from build123d import *

# Parameters (mm, degrees)
CHANFREIN1_SIZE                                = 0.5
FRAISAGE_POUR_VIS_T_TE_FRAIS_E_M31_D           = 3.2
FRAISAGE_POUR_VIS_T_TE_FRAIS_E_M31_CSINK_D     = 7.3
FRAISAGE_POUR_VIS_T_TE_FRAIS_E_M31_CSINK_ANGLE = 90
ENL_V_MAT_EXTRU_1_REACH                        = 94.326
ESQUISSE5_R                                    = 2.5


with BuildPart() as part:
    # Esquisse1 → Révolution1 (revolve)
    with BuildSketch(Plane.XY, mode=Mode.PRIVATE) as r_volution1_sk:
        Polygon((0, 10), (0, 20), (78, 20), (78, 30), (82, 30), (82, 17), (4, 17), (4, 10), align=None)
    revolve(r_volution1_sk.sketch.rotate(Axis((0, 0, 0), (1, 0, 0)), 90), axis=Axis((0, 0, 0), (1, 0, 0)))

    # Chanfrein1
    chanfrein1_edges = [part.edges().sort_by_distance(p)[0] for p in [
        (0, 0, -20),
        (78, 0, -30),
        (82, 0, -30),
        (82, 0, -17),
        (4, 0, -10),
    ]]
    chamfer(chanfrein1_edges, length=CHANFREIN1_SIZE)

    # Fraisage pour vis à tête fraisée M31 (through all)
    with Locations(Plane.ZY):
        with Locations((0, 13), (13, 0), (0, -13), (-13, 0)):
            CounterSinkHole(FRAISAGE_POUR_VIS_T_TE_FRAIS_E_M31_D / 2, FRAISAGE_POUR_VIS_T_TE_FRAIS_E_M31_CSINK_D / 2, counter_sink_angle=FRAISAGE_POUR_VIS_T_TE_FRAIS_E_M31_CSINK_ANGLE)

    # Esquisse5 → Enlèv. mat.-Extru.1 (cut, up to next)
    with BuildSketch(Plane(origin=(82, 0, 0), x_dir=(0, 0, -1), z_dir=(1, 0, 0)), mode=Mode.PRIVATE) as enl_v_mat_extru_1_sk1:
        with Locations((0, 25)):
            Circle(ESQUISSE5_R)
    enl_v_mat_extru_1_tool1 = extrude(enl_v_mat_extru_1_sk1.sketch, amount=-ENL_V_MAT_EXTRU_1_REACH, mode=Mode.PRIVATE) & part.part
    # Esquisse5 → Enlèv. mat.-Extru.1 (cut, up to next)
    with BuildSketch(Plane(origin=(82, 0, 0), x_dir=(0, 0, -1), z_dir=(1, 0, 0)), mode=Mode.PRIVATE) as enl_v_mat_extru_1_sk2:
        with Locations((25, 0)):
            Circle(ESQUISSE5_R)
    enl_v_mat_extru_1_tool2 = extrude(enl_v_mat_extru_1_sk2.sketch, amount=-ENL_V_MAT_EXTRU_1_REACH, mode=Mode.PRIVATE) & part.part
    # Esquisse5 → Enlèv. mat.-Extru.1 (cut, up to next)
    with BuildSketch(Plane(origin=(82, 0, 0), x_dir=(0, 0, -1), z_dir=(1, 0, 0)), mode=Mode.PRIVATE) as enl_v_mat_extru_1_sk3:
        with Locations((-25, 0)):
            Circle(ESQUISSE5_R)
    enl_v_mat_extru_1_tool3 = extrude(enl_v_mat_extru_1_sk3.sketch, amount=-ENL_V_MAT_EXTRU_1_REACH, mode=Mode.PRIVATE) & part.part
    # Esquisse5 → Enlèv. mat.-Extru.1 (cut, up to next)
    with BuildSketch(Plane(origin=(82, 0, 0), x_dir=(0, 0, -1), z_dir=(1, 0, 0)), mode=Mode.PRIVATE) as enl_v_mat_extru_1_sk4:
        with Locations((0, -25)):
            Circle(ESQUISSE5_R)
    enl_v_mat_extru_1_tool4 = extrude(enl_v_mat_extru_1_sk4.sketch, amount=-ENL_V_MAT_EXTRU_1_REACH, mode=Mode.PRIVATE) & part.part
    add(enl_v_mat_extru_1_tool1.solids().sort_by_distance((82, 25, 0))[0], mode=Mode.SUBTRACT)
    add(enl_v_mat_extru_1_tool2.solids().sort_by_distance((82, 0, -25))[0], mode=Mode.SUBTRACT)
    add(enl_v_mat_extru_1_tool3.solids().sort_by_distance((82, 0, 25))[0], mode=Mode.SUBTRACT)
    add(enl_v_mat_extru_1_tool4.solids().sort_by_distance((82, -25, 0))[0], mode=Mode.SUBTRACT)


solid = part.part
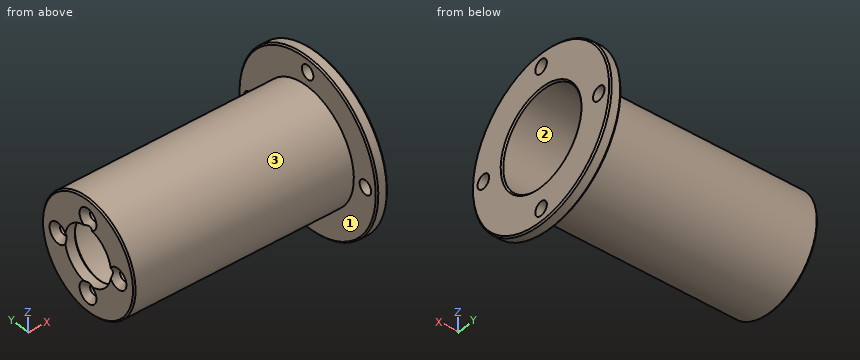
Here's how the part is built. I have some questions about the finished solid (model axes, mm). Face numbers are marked on the shaded views. Coordinates: 2 decimals unless noted, no trailing zeros. Loops run counter-clockwise (first coordinate to the right, second up) from the corner with the lowest first, then second, coordinate; pieces in that order, holes last.
1. I need wall thicknesses on L1, parallel to Y at x = 2, z = 0; L2, parallel to Y at x = 53, z = 0; L3, parallel to Y at x = 61, z = -9.5. Which ranges of each line are inside material? Lowest first, please.
2. If we mould it in two halves opening along Y, with no side actions, what happens to the marked faces 1, 2 and 3? For each: pulls with the +Y half, pulls with the -Y half, needs draft (parallel to the pull), parting line crosses it, or undercut.
3. Imagine slicing it at A-A, the plane z = 0. Count the separate pieces of the cut face and the enclosed holes in it, and give its area (3 significant figures).
4. Imagine slicing it at C-C, the plane x = 11. Please give me the cut outline in (y, z), and give its area (3 significant figures).
5. For P1, Ø5, axis at x = 28, z = 9.5, coming from the +Y side (3 decimals); P2, Ø3, axis at y = 25, z = 0, coming from the +X side; P3, Ø6, axis at x = 61, z = -20.5, coming from the -Y side; P4, Ø8, axis at x = 58.5, z = 16, coming from the +Y side, each with a flat end and sliding along its axis, tell me the tip position at first contact or that it passes through.
Taken from the geometry:
1. L1: y = -20 to -14.65, -11.35 to -10, 10 to 11.35, 14.65 to 20
1. L2: y = -20 to -17, 17 to 20
1. L3: y = -17.6 to -14.1, 14.1 to 17.6
2. face 1: needs draft
2. face 2: undercut
2. face 3: parting line crosses it
3. separate pieces: 6
3. enclosed holes: 0
3. area: 553 mm2
4. outline: circle Ø40 at (0, 0); hole circle Ø34 at (0, 0)
4. area: 349 mm2
5. P1: stops at y = 18.735
5. P2: passes through
5. P3: stops at y = -9.68
5. P4: stops at y = 16
